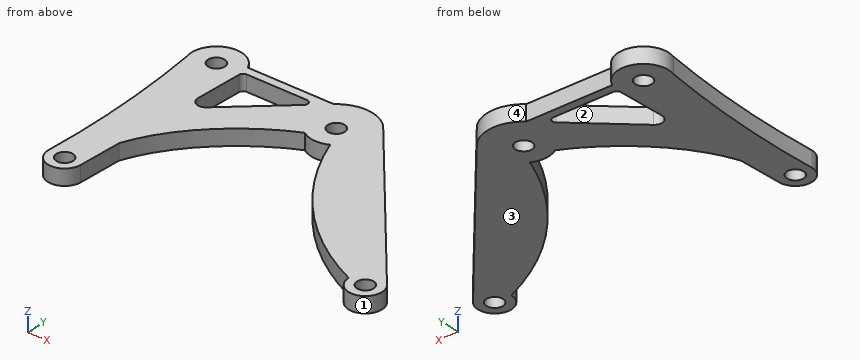
Autodesk Inventor part; units mm, degrees
ref_plane "YZ Plane" through (0, 0, 0) normal (1, 0, 0) x (0, 1, 0)
ref_plane "XZ Plane" through (0, 0, 0) normal (0, 1, 0) x (-1, 0, 0)
ref_plane "XY Plane" through (0, 0, 0) normal (0, 0, 1) x (1, 0, 0)
sketch "Sketch1" plane through (0, 0, 0) normal (0, 0, 1) x (1, 0, 0)
  line L0 (-110, 70) -> (110, 70) construction
  line L1 (110, 70) -> (110, -70) construction
  line L2 (110, -70) -> (-110, -70) construction
  line L3 (-110, -70) -> (-110, 70) construction
  circle A0 centre (-90, 55) radius 5
  circle A1 centre (-90, -55) radius 5
  circle A2 centre (90, -55) radius 5
  circle A3 centre (-10, 45) radius 5
  line L4 (-67, 0) -> (-42, 0) construction
  line L5 (-42, 0) -> (-42, -30) construction
  line L6 (-42, -30) -> (-67, -30) construction
  line L7 (-67, -30) -> (-67, 0) construction
  circle A4 centre (-54.5, -19) radius 10 construction
  arc A5 (-76.2883, 61.082) -> (-104.3936, 50.7781) centre (-90, 55) ccw
  arc A6 (-99.9402, -53.9078) -> (-80.0103, -55.4531) centre (-90, -55) ccw
  arc A7 (-100, -55) -> (-105, 55) centre (-644.4063, -24.6321) ccw
  line L8 (-78.8103, -29) -> (-67, 2.1947) construction
  line L9 (-67, 2.1947) -> (-37.7539, 24.0313) construction
  line L10 (-37.7539, 24.0313) -> (-18.5252, 32.6582) construction
  spline S0 degree 3 poles (-78.8103, -29) (-67, 2.1947) (-37.7539, 24.0313) (-18.5252, 32.6582) knots 1 1 1 1 2 2 2 2
  line L11 (-34.9568, 51.6958) -> (-68.1552, 21.4315)
  line L12 (-75.2957, 53.6513) -> (-76.519, 25.3424)
  line L13 (-78.8103, -29) -> (-80.0103, -55.4531)
  arc A8 (80, -55) -> (97.6304, -48.5365) centre (90, -55) ccw
  line L14 (5.2335, 60.5405) -> (97.6304, -48.5365)
  arc A9 (-2.7947, 31.8439) -> (80, -55) centre (141.6446, 86.6595) ccw
  arc A10 (-18.5252, 32.6582) -> (-2.7947, 31.8439) centre (-10, 45) ccw
  arc A11 (5.2335, 60.5405) -> (-24.6607, 61.082) centre (-10, 45) ccw
  arc A12 (-76.519, 25.3424) -> (-68.1552, 21.4315) centre (-71.5236, 25.1265) ccw
  line L15 (-76.2883, 61.082) -> (-24.6607, 61.082)
  line L16 (-72.7981, 56.0433) -> (-36.641, 56.0433)
  arc A13 (-72.7981, 56.0433) -> (-75.2957, 53.6513) centre (-72.7981, 53.5433) ccw
  arc A14 (-34.9568, 51.6958) -> (-36.641, 56.0433) centre (-36.641, 53.5433) ccw
  point P0 (0, 0)
  dimension "d1" = 70
  dimension "d2" = 70
  dimension "d3" = 110
  dimension "d4" = 110
  dimension "d5" = 10
  dimension "d6" = 10
  dimension "d7" = 10
  dimension "d8" = 10
  dimension "d9" = 55
  dimension "d10" = 55
  dimension "d11" = 55
  dimension "d12" = 180
  dimension "d13" = 90
  dimension "d15" = 10
  dimension "d16" = 45
  dimension "d17" = 42
  dimension "d18" = 30
  dimension "d19" = 0
  dimension "d20" = 25
  dimension "d21" = 20
  dimension "d25" = 19
  dimension "d26" = 12.5
  dimension "d67" = 90
  dimension "d68" = 30
  dimension "d70" = 20
  dimension "d71" = 20
  dimension "d74" = 10
  dimension "d75" = 5
  dimension "d76" = 5
extrude "Extrusion6" add sketch "Sketch1" along normal blind 9.4 contours L15 A11 L14 A8 A9 A10 S0 L13 A6 A7 A5 | A7 A5
equation "\"d26\" = 0.5 * d20"
properties part number "Bracket Concept MK9"
For this review, take the finished solid that the model builds, in its own axes (mm). Face numbers are marked on the shaded views. Give positions to 0.01 mm unless a question says otherwise; leave off trailing zeros. Loops run counter-clockwise (first coordinate to the right, second up) from the corner with the lowest first, then second, coordinate; pieces in that order, holes last. Notation, with made-up numbers: M 55.25,40.5 L 112.25,40.5 A19 cw 112.25,45.5 Z; hole C -19,89.25 d8. An arc over 180 degrees is marked long. Answer as a JSON object with one key per item and string values. Group by question number.
Q1. Add section C-C on y = -52. Give the boundary of the cut face in (x, z), and give its area (3 significant figures).
Q2. Add section A-A on x = -10. Give the boundary of the cut face in (y, z), and give its area (3 significant figures).
Q3. Insertion check: P1, Ø1.5, axis at x = -29.5, z = 1.5, coming from the +Y side; P2, Ø1, axis at y = -38.5, z = 6, coming from the +X side; P3, Ø5, axis at x = 32, z = 4, coming from the +Y side. Each pin has a flat end and moves straight along its axis. Give the tip position at first contact, or say it passes through.
Q4. For probe 1 along Y at (x, z) = (-90, 2); probe 2 along X at (y, z) = (-59, 4.75); probe 3 along X at (y, z) = (22, 3.75), list the stretches that pass through material, from the lowest coordinate up. Write a range as [from, to].
Q5. Mouldability with a two-part tool opening along Y and no side actions: class the marked faces 1, 2, 3 and 4 as +Y half, -Y half, draft (parallel to the pull), parting line (faces both ways), or undercut.
Q6. Add section D-D on z = 3.25. Give the number of separate pieces and of enclosed holes in the cut face, and give its area (3 significant figures).
Q7. Add section B-B on x = -90. Give the boundary of the cut face in (y, z).
Checked values:
{
 "1": {"outline": "M -99.84,0 L -94,0 L -94,9.4 L -99.84,9.4 Z; M -86,0 L -79.85,0 L -79.85,9.4 L -86,9.4 Z; M 73.52,0 L 86,0 L 86,9.4 L 73.52,9.4 Z; M 94,0 L 99.54,0 L 99.54,9.4 L 94,9.4 Z", "area": "282 mm²"},
 "2": {"outline": "M 30,0 L 40,0 L 40,9.4 L 30,9.4 Z; M 50,0 L 66.76,0 L 66.76,9.4 L 50,9.4 Z", "area": "252 mm²"},
 "3": {"P1": "y = 61.08", "P2": "x = 89.55", "P3": "y = 31.89"},
 "4": {"probe 1": "[-65, -60], [-50, 50], [60, 70]", "probe 2": "[-99.17, -93], [-87, -80.83], [80.83, 87], [93, 99.17]", "probe 3": "[-101.15, -75.43], [-67.53, -36.99], [1.34, 37.88]"},
 "5": {"face 1": "parting line", "face 2": "undercut", "face 3": "draft", "face 4": "+Y half"},
 "6": {"separate pieces": "1", "enclosed holes": "5", "area": "9,450 mm²"},
 "7": {"outline": "M -65,0 L -60,0 L -60,9.4 L -65,9.4 Z; M -50,0 L 50,0 L 50,9.4 L -50,9.4 Z; M 60,0 L 70,0 L 70,9.4 L 60,9.4 Z"}
}
